```python
from build123d import *

# Parameters (mm, degrees)
F0_W     = 127
F0_H     = 127
F1_DEPTH = 321.1322
F2_R     = 170.815
F3_DEPTH = 66.04
F4_R     = 114.3
F5_DEPTH = 119.38
F6_R     = 25.4
F7_DEPTH = 50.8
F8_R     = 12.7
F9_DEPTH = 224.79


with BuildPart() as f1:
    # F0 (on Front) → F1 (new body)
    with BuildSketch(Plane.XZ):
        Rectangle(F0_W, F0_H)
    extrude(amount=-F1_DEPTH)

    # F2 (on Front) → F3 (join, symmetric)
    with BuildSketch(Plane.XZ):
        Circle(F2_R)
    extrude(amount=F3_DEPTH, both=True)

    # F4 (on face) → F5 (join)
    with BuildSketch(Plane.XZ.offset(66.04)):
        Circle(F4_R)
    extrude(amount=F5_DEPTH)

    # F6 (on face) → F7 (join)
    with BuildSketch(Plane.XZ.offset(185.42)):
        Circle(F6_R)
    extrude(amount=F7_DEPTH)

    # F8 (on Right) → F9 (join, symmetric)
    with BuildSketch(Plane.YZ):
        Circle(F8_R)
    extrude(amount=F9_DEPTH, both=True)


solid = f1.part
```
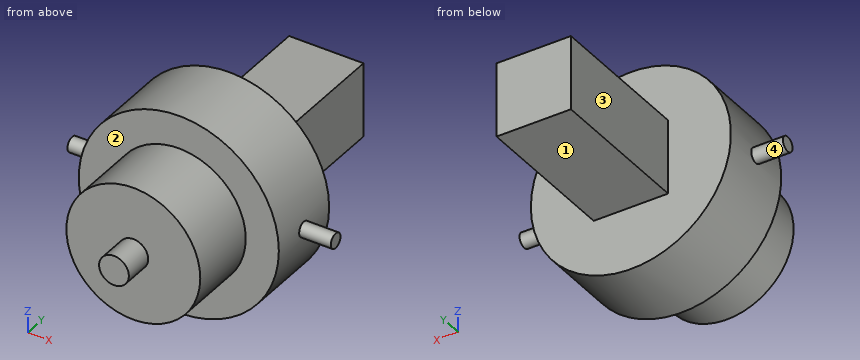
Here's how the part is built. I have some questions about the finished solid (model axes, mm). Face numbers are marked on the shaded views. A direction names the side the tool comes from. Coordinates: 2 decimals unless noted, no trailing zeros. Loops run counter-clockwise (first coordinate to the right, second up) from the corner with the lowest first, then second, coordinate; pieces in that order, holes last. Notation, with made-up numbers: (18.5, -13) -> (58.5, -13) arc R30 cw to (58.5, 25) -> close; hole circle Ø7 at (56, -8.75). An arc over 180 degrees is marked (long way). Return JSON: item names as keys, results as strings.
1) If we section it at C-C, the plane x = 88: Write out the boundary of the cut face in (y, z), then the cut area to 3 significant figures.
Results below:
{"outline": "(-185.42, -72.94) -> (-66.04, -72.94) -> (-66.04, -146.4) -> (66.04, -146.4) -> (66.04, 146.4) -> (-66.04, 146.4) -> (-66.04, 72.94) -> (-185.42, 72.94) -> close", "area": "56,100 mm²"}
2) For the marked faces 1, 2, 3 and 4, which set-ups out of +Z, -Z, +X, -X, +Y, -Y let a thin tool reach every point of the face, with its end or its side?
Results below:
{"face 1": "-Z, +X, -X, +Y", "face 2": "-Y", "face 3": "+Z, -Z, -X, +Y", "face 4": "-X"}
3) If we section it at B-B, the plane z = 0: Write out the boundary of the cut face in (x, y) (3 decimals), then the cut area to 3 significant figures.
Results below:
{"outline": "(-224.79, -12.7) -> (-170.815, -12.7) -> (-170.815, -66.04) -> (-114.3, -66.04) -> (-114.3, -185.42) -> (-25.4, -185.42) -> (-25.4, -236.22) -> (25.4, -236.22) -> (25.4, -185.42) -> (114.3, -185.42) -> (114.3, -66.04) -> (170.815, -66.04) -> (170.815, -12.7) -> (224.79, -12.7) -> (224.79, 12.7) -> (170.815, 12.7) -> (170.815, 66.04) -> (63.5, 66.04) -> (63.5, 321.132) -> (-63.5, 321.132) -> (-63.5, 66.04) -> (-170.815, 66.04) -> (-170.815, 12.7) -> (-224.79, 12.7) -> close", "area": "110,000 mm²"}
4) I need wall thicknesses on line 1 (Y direction, x = 57.5, z = -5); line 2 (X direction, y = 235, z = 44.5); line 3 (Y direction, x = 85, z = 85). Which ranges of each line are inside material? Lowest first, please. Write a range as from..to.
Results below:
{"line 1": "-185.42..321.13", "line 2": "-63.5..63.5", "line 3": "-66.04..66.04"}
5) If we section it at A-A, the plane y = 0: Write out the boundary of the cut face in (x, z) (3 decimals).
Results below:
{"outline": "(-224.79, -12.7) -> (-170.342, -12.7) arc R170.815 ccw to (170.342, -12.7) -> (224.79, -12.7) -> (224.79, 12.7) -> (170.342, 12.7) arc R170.815 ccw to (-170.342, 12.7) -> (-224.79, 12.7) -> close"}
6) Will these pins go through, and if not, where does the flat tip stop? pin 1 (2 mm diameter, centred on y = 196, z = -49.5, fed in from +X); pin 2 (8 mm diameter, centred on x = 22, y = -118, fed in from +Z); pin 3 (8 mm diameter, centred on x = -164.5, z = -25.5, fed in from +Y).
Results below:
{"pin 1": "x = 63.5", "pin 2": "z = 112.87", "pin 3": "y = 66.04"}
7) If we section it at D-D, the plane z = -43: Write out the boundary of the cut face in (x, y), then the cut area to 3 significant figures.
Results below:
{"outline": "(-165.31, -66.04) -> (-105.9, -66.04) -> (-105.9, -185.42) -> (105.9, -185.42) -> (105.9, -66.04) -> (165.31, -66.04) -> (165.31, 66.04) -> (63.5, 66.04) -> (63.5, 321.13) -> (-63.5, 321.13) -> (-63.5, 66.04) -> (-165.31, 66.04) -> close", "area": "101,000 mm²"}
